For this review, take the finished solid that the model builds, in its own axes (mm). Face numbers are marked on the shaded views. A direction names the side the tool comes from. Give positions to 0.01 mm unless a question says otherwise; leave off trailing zeros. Order: outer loops, then holes, each group sorted by start corner. A loop starts at its lowest first (then second) coordinate and runs counter-clockwise, first axis right, second up.
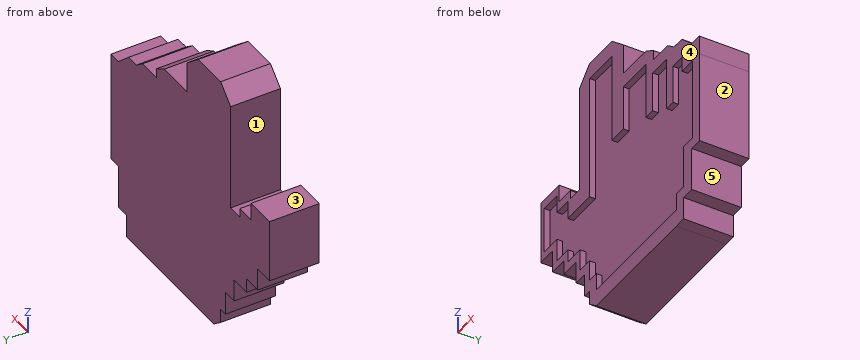
from build123d import *

# Parameters (mm, degrees)
F1_DEPTH = 11.684
F2_DEPTH = 13.208


# Not quite as in the source:
# - a feature names something its author has since deleted; it is built from what else it names


with BuildPart() as f1:
    # F0 (on Front) → F1 (new body)
    with BuildSketch(Plane.XZ):
        Polygon((9.8076034337, -4.2564473115), (0, -4.2564473115), (0, -28.2072033733), (0, -37.9272252321), (-4.4246674515, -37.9272252321), (-9.569064714, -37.9272252321), (-9.569064714, -33.0672143027), (-14.3852122128, -33.0672143027), (-14.3852122128, -28.3846426755), (-19.9310798198, -28.3846426755), (-19.9310798198, -40.7246947289), (-14.3852122128, -40.7246947289), (-14.3852122128, -46.85433954), (-9.569064714, -46.85433954), (-9.569064714, -50.3569915891), (-4.1691423394, -50.3569915891), (-4.1691423394, -56.1947450042), (0, -56.1947450042), (0, -61.7406144738), (2.9821074568, -61.7406144738), (2.9821074568, -66.3378462195), (38.154579699, -66.3378462195), (38.154579699, -61.7406144738), (41.2194021046, -61.7406144738), (41.2194021046, -50.3569915891), (45.0411513448, -50.3569915891), (45.0411513448, -28.3846426755), (40.5284799635, -28.3846426755), (40.5284799635, -24.3923105299), (36.5364998579, -24.3923105299), (36.5364998579, -34.6322879195), (33.7594784796, -34.6322879195), (33.7594784796, -24.3923105299), (33.7594784796, -20.5733645707), (27.6847239584, -20.5733645707), (27.6847239584, -31.3338786364), (24.7341338545, -31.3338786364), (24.7341338545, -20.5733645707), (24.7341338545, -16.2325797137), (14.8409679532, -16.2325797137), (14.8409679532, -28.2087121159), (9.8076034337, -28.2087121159), align=None)
    extrude(amount=F1_DEPTH)

    # F0 (on Front) → F2 (join)
    with BuildSketch(Plane.XZ):
        Polygon((9.8076034337, 0), (0, 0), (-4.4246674515, -4.2564473115), (-4.4246674515, -28.2072033733), (-4.4246674515, -33.0672143027), (-8.441273123, -33.0877043307), (-8.441273123, -30.6703820825), (-13.3577445522, -30.6703820825), (-13.3577445522, -26.0001793504), (-21.4487463236, -26.0001793504), (-21.4487463236, -42.8537763655), (-16.2677373737, -42.8537763655), (-16.2677373737, -48.8393343985), (-11.3371098414, -48.8393343985), (-11.3371098414, -52.6647716761), (-5.9138466604, -52.6647716761), (-5.9138466604, -58.6375892162), (-2.1712374873, -58.6375892162), (-2.1712374873, -64.7857561707), (0, -64.7857561707), (0, -68.5636028647), (2.9821074568, -70.9350779653), (38.154579699, -70.9350779653), (41.2194021046, -70.8393231034), (41.2194021046, -64.7857561707), (44.7839312255, -64.7857561707), (44.7839312255, -61.7406144738), (44.7839312255, -53.1140379608), (48.2247062027, -53.1140379608), (48.2247062027, -50.3569915891), (48.2247062027, -28.3846426755), (48.131018877, -23.2601258904), (44.8739007115, -23.2601258904), (40.4558517039, -19.210241735), (37.0195880532, -19.210241735), (34.1969430447, -17.0012172312), (28.0607584864, -17.0012172312), (28.0607584864, -14.4240194932), (24.7341338545, -12.4151380733), (14.8409679532, -12.4151380733), (14.8409679532, -4.2564473115), align=None)
        Polygon((0, -28.2072033733), (0, -4.2564473115), (9.8076034337, -4.2564473115), (9.8076034337, -28.2087121159), (14.8409679532, -28.2087121159), (14.8409679532, -16.2325797137), (24.7341338545, -16.2325797137), (24.7341338545, -20.5733645707), (24.7341338545, -31.3338786364), (27.6847239584, -31.3338786364), (27.6847239584, -20.5733645707), (33.7594784796, -20.5733645707), (33.7594784796, -24.3923105299), (33.7594784796, -34.6322879195), (36.5364998579, -34.6322879195), (36.5364998579, -24.3923105299), (40.5284799635, -24.3923105299), (40.5284799635, -28.3846426755), (45.0411513448, -28.3846426755), (45.0411513448, -50.3569915891), (41.2194021046, -50.3569915891), (41.2194021046, -61.7406144738), (38.154579699, -61.7406144738), (38.154579699, -66.3378462195), (2.9821074568, -66.3378462195), (2.9821074568, -61.7406144738), (0, -61.7406144738), (0, -56.1947450042), (-4.1691423394, -56.1947450042), (-4.1691423394, -50.3569915891), (-9.569064714, -50.3569915891), (-9.569064714, -46.85433954), (-14.3852122128, -46.85433954), (-14.3852122128, -40.7246947289), (-19.9310798198, -40.7246947289), (-19.9310798198, -28.3846426755), (-14.3852122128, -28.3846426755), (-14.3852122128, -33.0672143027), (-9.569064714, -33.0672143027), (-9.569064714, -37.9272252321), (-4.4246674515, -37.9272252321), (0, -37.9272252321), align=None, mode=Mode.SUBTRACT)
    extrude(amount=F2_DEPTH)


solid = f1.part
1) We need section B-B on z = -45. Give the boundary of the cut face in (x, y).
Answer sheet:
outline: (-16.27, -13.21) - (-14.39, -13.21) - (-14.39, -11.68) - (45.04, -11.68) - (45.04, -13.21) - (48.22, -13.21) - (48.22, 0) - (-16.27, 0) - close
2) To check wall thickness, follow line 1 (X direction, y = -9.5, z = -29); line 2 (Y direction, x = 6.5, z = -58); line 3 (X direction, y = -11.5, z = -5). State the ranges of each line that lie inside material, in increasing order.
Answer sheet:
line 1: x = -21.45 to -13.36, -4.42 to 48.22
line 2: y = -11.68 to 0
line 3: x = -4.42 to 14.84
3) Clearance check with flat-ended pins moving along their axes: pin 1 (12 mm diameter, centred on x = 6.5, z = -41.5, fed in from -Y); pin 2 (1.7 mm diameter, centred on x = -1.5, y = -5.5, fed in from -Z); pin 3 (1.2 mm diameter, centred on x = -3, y = -12.5, fed in from -Z). State where each tip first meets the part, or that it passes through.
Answer sheet:
pin 1: stops at y = -11.68
pin 2: stops at z = -64.79
pin 3: stops at z = -58.64
4) We need section A-A on x = 18.5. Give the boundary of the cut face in (y, z).
Answer sheet:
outline: (-13.21, -70.94) - (0, -70.94) - (0, -12.42) - (-13.21, -12.42) - (-13.21, -16.23) - (-11.68, -16.23) - (-11.68, -66.34) - (-13.21, -66.34) - close
5) Tool access review of the marked faces 1, 2, 3, 4 and 5: name each direction out of +Z, -Z, +X, -X, +Y, -Y from which nothing blocks a thin tool from reaching the whole face with its end or side.
Answer sheet:
face 1: +Z, +Y, -Y
face 2: +Z, -Z, +X, +Y, -Y
face 3: +Z, -X, +Y, -Y
face 4: +Z, -Z, +X, -X, -Y
face 5: -Z, +X, +Y, -Y
